```python
from build123d import *

# Parameters (mm, degrees)
SKETCH1_R           = 5
SKETCH1_R_2         = 4.5
BOSS_EXTRUDE1_DEPTH = 50.87650029
SKETCH2_R           = 6
SKETCH2_R_2         = 2.5
BOSS_EXTRUDE2_DEPTH = 1
SKETCH3_R           = 6
SKETCH3_R_2         = 2.5
BOSS_EXTRUDE3_DEPTH = 1


with BuildPart() as part:
    # Sketch1 → Boss-Extrude1 (new body)
    with BuildSketch(Plane.XY):
        Circle(SKETCH1_R)
        Circle(SKETCH1_R_2, mode=Mode.SUBTRACT)
    extrude(amount=BOSS_EXTRUDE1_DEPTH)

    # Sketch2 → Boss-Extrude2 (add)
    with BuildSketch(Plane(origin=(0, 0, 0), x_dir=(-1, 0, 0), z_dir=(0, 0, -1))):
        Circle(SKETCH2_R)
        Circle(SKETCH2_R_2, mode=Mode.SUBTRACT)
    extrude(amount=BOSS_EXTRUDE2_DEPTH)

    # Sketch3 → Boss-Extrude3 (add)
    with BuildSketch(Plane.XY.offset(50.87650029)):
        Circle(SKETCH3_R)
        Circle(SKETCH3_R_2, mode=Mode.SUBTRACT)
    extrude(amount=BOSS_EXTRUDE3_DEPTH)


solid = part.part
```
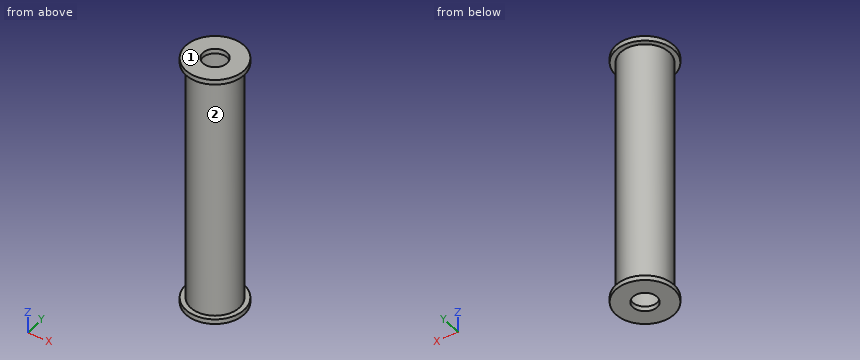
Here's how the part is built. I have some questions about the finished solid (model axes, mm). Face numbers are marked on the shaded views. A direction names the side the tool comes from. Coordinates: 2 decimals unless noted, no trailing zeros. Write each loop counter-clockwise with the first axis right and the second up, starting at its lowest first coordinate (ties: lowest second). Pieces come first, ordered by that corner, then holes. Notation, with made-up numbers: (29, -15) - (66, -15) arc R27 ccw to (66, 18) - close; hole circle Ø2 at (10, -12.75). An arc over 180 degrees is marked (long way). One line per item, written item: value.
1) I'm going to push flat-ended pins straight in: P1, Ø4, axis at y = 0.5, z = 16.5, coming from the -X side; P2, Ø4, axis at y = 4, z = 40, coming from the +X side; P3, Ø6, axis at x = -2.5, z = 28.5, coming from the +Y side; P4, Ø6.5, axis at x = 0, y = 0, coming from the +Z side. Where does each tip first touch, or does it pass through?
Model answer:
P1: stops at x = -5
P2: stops at x = 4.58
P3: stops at y = 5
P4: stops at z = 51.88
2) On a 3-axis mill with a long thin cutter (end or side, diameter ignored), from which of +Z, -Z, +X, -X, +Y, -Y can I reach the whole of each face in a straight line? I mean the marked faces 1 and 2. Say none if no direction works.
Model answer:
face 1: +Z, +X, -X, +Y, -Y
face 2: none
3) Suppose I cut it at B-B on y = 0.5. Write out the boundary of the cut face in (x, z).
Model answer:
outline: (-5.98, -1) - (-2.45, -1) - (-2.45, 0) - (-4.47, 0) - (-4.47, 50.88) - (-2.45, 50.88) - (-2.45, 51.88) - (-5.98, 51.88) - (-5.98, 50.88) - (-4.97, 50.88) - (-4.97, 0) - (-5.98, 0) - close; (2.45, -1) - (5.98, -1) - (5.98, 0) - (4.97, 0) - (4.97, 50.88) - (5.98, 50.88) - (5.98, 51.88) - (2.45, 51.88) - (2.45, 50.88) - (4.47, 50.88) - (4.47, 0) - (2.45, 0) - close
4) I need wall thicknesses on line 1 along Z through (x, y) = (-3.5, 0.5); line 2 along Y through (x, z) = (0, 51.25); line 3 along Y through (x, z) = (0, 35.5). Which ranges of each line are inside material? Lowest first, please.
Model answer:
line 1: z = -1 to 0, 50.88 to 51.88
line 2: y = -6 to -2.5, 2.5 to 6
line 3: y = -5 to -4.5, 4.5 to 5
5) Suppose I cut it at A-A on x = 0. Write out the boundary of the cut face in (y, z), and give its area (3 significant figures).
Model answer:
outline: (-6, -1) - (-2.5, -1) - (-2.5, 0) - (-4.5, 0) - (-4.5, 50.88) - (-2.5, 50.88) - (-2.5, 51.88) - (-6, 51.88) - (-6, 50.88) - (-5, 50.88) - (-5, 0) - (-6, 0) - close; (2.5, -1) - (6, -1) - (6, 0) - (5, 0) - (5, 50.88) - (6, 50.88) - (6, 51.88) - (2.5, 51.88) - (2.5, 50.88) - (4.5, 50.88) - (4.5, 0) - (2.5, 0) - close
area: 64.9 mm²
6) Suppose I cut it at D-D on x = 3. Write out the boundary of the cut face in (y, z).
Model answer:
outline: (-5.2, -1) - (5.2, -1) - (5.2, 0) - (4, 0) - (4, 50.88) - (5.2, 50.88) - (5.2, 51.88) - (-5.2, 51.88) - (-5.2, 50.88) - (-4, 50.88) - (-4, 0) - (-5.2, 0) - close; hole (-3.35, 0) - (3.35, 0) - (3.35, 50.88) - (-3.35, 50.88) - close
7) Suppose I cut it at C-C on y = 3.75. Write out the boundary of the cut face in (x, z).
Model answer:
outline: (-4.68, -1) - (4.68, -1) - (4.68, 0) - (3.31, 0) - (3.31, 50.88) - (4.68, 50.88) - (4.68, 51.88) - (-4.68, 51.88) - (-4.68, 50.88) - (-3.31, 50.88) - (-3.31, 0) - (-4.68, 0) - close; hole (-2.49, 0) - (2.49, 0) - (2.49, 50.88) - (-2.49, 50.88) - close
